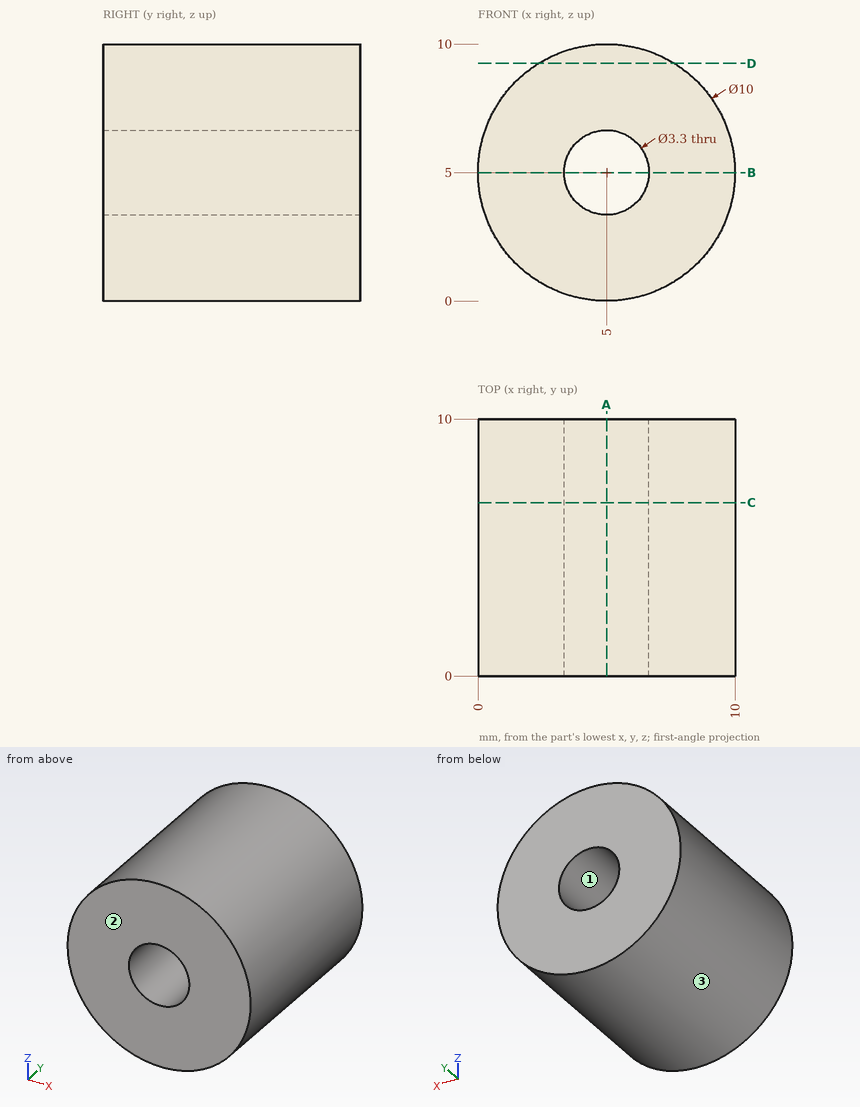
The figure shows three views and two pictorial views of one solid part (mm, origin at its lowest corner). Answer the questions. Coordinates: 2 decimals unless noted, no trailing zeros. Loops run counter-clockwise (first coordinate to the right, second up) from the corner with the lowest first, then second, coordinate; pieces in that order, holes last.
(1) The mould has two halves that part along X. Classify the marked faces 1, 2 and 3: released by +X, released by -X, zero draft, split by the parting line, or undercut.
Solution:
face 1: undercut
face 2: zero draft
face 3: split by the parting line
(2) Consider line 1 along Z through (x, y) = (3.5, 5.5); line 2 along X through (y, z) = (8.5, 3.75); line 3 along X through (y, z) = (7.75, 5.75). Determine where each line is inside the solid, lowest interval first.
Solution:
line 1: z = 0.23 to 4.31, 5.69 to 9.77
line 2: x = 0.16 to 3.92, 6.08 to 9.84
line 3: x = 0.06 to 3.53, 6.47 to 9.94
(3) The part is cut by section B-B (z = 5). Determine the outline of the cut face in (x, y).
Solution:
outline: (0, 0) - (3.35, 0) - (3.35, 10) - (0, 10) - close; (6.65, 0) - (10, 0) - (10, 10) - (6.65, 10) - close
(4) The part is cut by section D-D (z = 9.25). Determine the outline of the cut face in (x, y).
Solution:
outline: (2.37, 0) - (7.63, 0) - (7.63, 10) - (2.37, 10) - close
(5) Flat-ended cylindrical pins translate along their axes: pin 1 Ø6 at (x, y) = (8.5, 5.5) entering from -Z; pin 2 Ø5 at (y, z) = (7, 1.5) entering from +X; pin 3 Ø1.5 at (x, y) = (8, 8.5) entering from -Z. Find the tip coordinate at first contact, or state that the pin passes through.
Solution:
pin 1: stops at z = 0.03
pin 2: stops at x = 9.9
pin 3: stops at z = 0.53
(6) The part is cut by section C-C (y = 6.75). Determine the outline of the cut face in (x, z).
Solution:
outline: circle Ø10 at (5, 5); hole circle Ø3.3 at (5, 5)
(7) The part is cut by section A-A (x = 5). Determine the outline of the cut face in (y, z), and give its area (3 significant figures).
Solution:
outline: (0, 0) - (10, 0) - (10, 3.35) - (0, 3.35) - close; (0, 6.65) - (10, 6.65) - (10, 10) - (0, 10) - close
area: 67.0 mm2
